Source: CAD feature listing. Evaluate the final solid. Frame: model axes, mm. Face numbers are marked on the shaded views. A direction names the side the tool comes from. Coordinates: 2 decimals unless noted, no trailing zeros. Order: outer loops, then holes, each group sorted by start corner. A loop starts at its lowest first (then second) coordinate and runs counter-clockwise, first axis right, second up. Notation, with made-up numbers: (63, -40) -> (108, -40) arc R20 cw to (108, -26) -> close; hole circle Ø6 at (-12.5, 37.5). An arc over 180 degrees is marked (long way). Put each result on its own line as item: value.
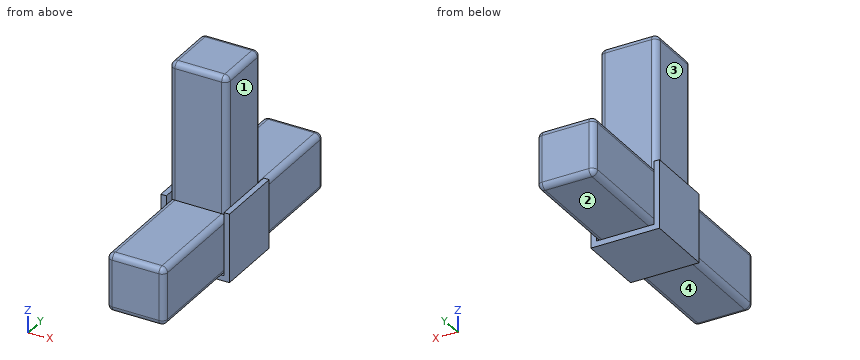
from build123d import *

# Parameters (mm, degrees)
F0_W      = 21
F0_H      = 21
F1_DEPTH  = 100
F2_W      = 21
F2_H      = 21
F3_DEPTH  = 50
F4_R      = 2
F6_DEPTH  = 2
F7_W      = 25
F7_H      = 25
F8_DEPTH  = 2
F9_W      = 25
F9_H      = 25
F10_DEPTH = 2


with BuildPart() as f1:
    # F0 (on Front) → F1 (new body)
    with BuildSketch(Plane.XZ):
        Rectangle(F0_W, F0_H)
    extrude(amount=F1_DEPTH)

    # F2 (on face) → F3 (join)
    with BuildSketch(Plane.XY.offset(10.5)):
        with Locations((0, -50)):
            Rectangle(F2_W, F2_H)
    extrude(amount=F3_DEPTH)

    # F4
    f4_edges = [f1.edges().sort_by_distance(p)[0] for p in [
        (-10.5, -19.75, 10.5),
        (-10.5, -80.25, 10.5),
        (10.5, -80.25, 10.5),
        (10.5, -19.75, 10.5),
        (10.5, -50, -10.5),
        (-10.5, -50, -10.5),
        (-10.5, -100, 0),
        (0, -100, 10.5),
        (10.5, -100, 0),
        (0, -100, -10.5),
        (10.5, 0, 0),
        (0, 0, 10.5),
        (-10.5, 0, 0),
        (0, 0, -10.5),
        (-10.5, -60.5, 35.5),
        (10.5, -60.5, 35.5),
        (0, -60.5, 60.5),
        (10.5, -50, 60.5),
        (-10.5, -50, 60.5),
        (0, -39.5, 60.5),
        (10.5, -39.5, 35.5),
        (-10.5, -39.5, 35.5),
    ]]
    fillet(f4_edges, radius=F4_R)

    # F5 (on face) → F6 (join)
    with BuildSketch(Plane(origin=(-10.5, 0, 0), x_dir=(0, -1, 0), z_dir=(-1, 0, 0))):
        Polygon((62.5, 12.5), (37.5, 12.5), (37.5, 10.5), (37.5, -12.5), (62.5, -12.5), (62.5, 10.5), align=None)
    extrude(amount=F6_DEPTH)

    # F7 (on face) → F8 (join)
    with BuildSketch(Plane.YZ.offset(10.5)):
        with Locations((-50, 0)):
            Rectangle(F7_W, F7_H)
    extrude(amount=F8_DEPTH)

    # F9 (on face) → F10 (join)
    with BuildSketch(Plane(origin=(0, 0, -10.5), x_dir=(1, 0, 0), z_dir=(0, 0, -1))):
        with Locations((0, 50)):
            Rectangle(F9_W, F9_H)
    extrude(amount=F10_DEPTH)


solid = f1.part
1. Cut plane A-A on x = 4. Output: boundary loops of the cut face in (y, z).
Numbers:
outline: (-100, -8.5) arc R2 ccw to (-98, -10.5) -> (-62.5, -10.5) -> (-62.5, -12.5) -> (-37.5, -12.5) -> (-37.5, -10.5) -> (-2, -10.5) arc R2 ccw to (0, -8.5) -> (0, 8.5) arc R2 ccw to (-2, 10.5) -> (-39.5, 10.5) -> (-39.5, 58.5) arc R2 ccw to (-41.5, 60.5) -> (-58.5, 60.5) arc R2 ccw to (-60.5, 58.5) -> (-60.5, 10.5) -> (-98, 10.5) arc R2 ccw to (-100, 8.5) -> close
2. Cut plane C-C on z = 50.5. Output: boundary loops of the cut face in (x, y), plus the area to 3 significant figures.
Numbers:
outline: (-10.5, -58.5) arc R2 ccw to (-8.5, -60.5) -> (8.5, -60.5) arc R2 ccw to (10.5, -58.5) -> (10.5, -41.5) arc R2 ccw to (8.5, -39.5) -> (-8.5, -39.5) arc R2 ccw to (-10.5, -41.5) -> close
area: 438 mm2
3. Ray query, line 1 along X through (y, z) = (-49, 39); line 2 along Y through (x, z) = (2.5, 51.5). Return the intervals inside material, ascending.
Numbers:
line 1: x = -10.5 to 10.5
line 2: y = -60.5 to -39.5
4. Set-up query: the marked faces 1, 2, 3 and 4. Return all of +Z, -Z, +X, -X, +Y, -Y with unobstructed straight access to the full face (end or side cutting, diameter ignored); none if empty.
Numbers:
face 1: +Z, +X, +Y, -Y
face 2: -Z, +X, -X, +Y
face 3: +Z, -X, +Y, -Y
face 4: -Z, +X, -X, -Y
5. Cut plane B-B on y = -72. Output: boundary loops of the cut face in (x, z).
Numbers:
outline: (-10.5, -8.5) arc R2 ccw to (-8.5, -10.5) -> (8.5, -10.5) arc R2 ccw to (10.5, -8.5) -> (10.5, 8.5) arc R2 ccw to (8.5, 10.5) -> (-8.5, 10.5) arc R2 ccw to (-10.5, 8.5) -> close
6. First-contact query: pin 1 (18.5 mm diameter, centred on y = -26, z = 2, fed in from -X); pin 2 (10 mm diameter, centred on y = -55.5, z = 40.5, fed in from +X); pin 3 (4 mm diameter, centred on x = 8, z = 39, fed in from +Y). Flat tips, straight axial feed; report the tip coordinate or a pass-through.
Numbers:
pin 1: stops at x = -10.5
pin 2: stops at x = 10.5
pin 3: stops at y = -39.5
